Build history of the part. All positions in model axes, mm. A direction names the side the tool comes from. Give positions to 0.01 mm unless a question says otherwise; leave off trailing zeros. Loops run counter-clockwise (first coordinate to the right, second up) from the corner with the lowest first, then second, coordinate; pieces in that order, holes last.
1) Band-saw the part on B-B on z = -75. List the corners of the cut face in (x, y).
2) Two-plate mould, pull along Y, no slides. Class faces 1 (the flat face through (3, -2, -100)), 2 (the flat face through (2.96, 119.47, 83.25)), 3 (the flat face through (3, -150, 1)): +Y half, -Y half, draft (parallel to the pull), parting line (faces both ways), or undercut.
3) 3-axis set-ups, long thin cutter, end or side, ignore diameter. For faces 4 (the flat face through (2.96, 47.33, 27.95)), 5 (the flat face through (0, 2, 1)): which of +Z, -Z, +X, -X, +Y, -Y reach the whole face in a straight line?
4) Band-saw the part on A-A on x = 1.1. List the corners of the cut face in (y, z), then the cut area to 3 significant figures.
5) Wall check: line 1 (Z direction, x = 1.8, y = 38); line 2 (Y direction, x = 0.8, z = -15); line 3 (Z direction, x = 2.2, y = 129.5). Give the ranges that are in metal, low to high.
```python
from build123d import *

# Parameters (mm, degrees)
SKETCH_1_W      = 200
SKETCH_1_H      = 300
EXTRUDE_1_DEPTH = 6


with BuildPart() as part:
    # Эскиз1 → Бобышка-Вытянуть1 (new body)
    with BuildSketch(Plane(origin=(0, 0, 0), x_dir=(0, 0, -1), z_dir=(1, 0, 0))):
        Rectangle(SKETCH_1_W, SKETCH_1_H)
        Polygon((-91.932327425, 143.306818051), (-96.924629192, 139.978616874), (-69.18961938, 98.376102157), (-64.197317614, 101.704303335), align=None, mode=Mode.SUBTRACT)
        Polygon((-19.26660172, 23.491575667), (-14.274299954, 26.819776844), (-42.009309765, 68.422291561), (-47.001611531, 65.094090384), align=None, mode=Mode.SUBTRACT)
        Polygon((19.26660172, 23.491575667), (47.001611531, 65.094090384), (42.009309765, 68.422291561), (14.274299954, 26.819776844), align=None, mode=Mode.SUBTRACT)
        Polygon((96.924629192, 139.978616874), (69.18961938, 98.376102157), (64.197317614, 101.704303335), (91.932327425, 143.306818051), align=None, mode=Mode.SUBTRACT)
    extrude(amount=EXTRUDE_1_DEPTH)


solid = part.part
```
Findings below:
1. outline: (0, -150) - (6, -150) - (6, 107.09) - (0, 107.09) - close; (0, 117.91) - (6, 117.91) - (6, 150) - (0, 150) - close
2. face 1: draft
2. face 2: undercut
2. face 3: -Y half
3. face 4: +X, -X
3. face 5: +Z, -Z, -X, +Y, -Y
4. outline: (-150, -100) - (150, -100) - (150, 100) - (-150, 100) - close; hole (23.49, -19.27) - (65.09, -47) - (68.42, -42.01) - (26.82, -14.27) - close; hole (23.49, 19.27) - (26.82, 14.27) - (68.42, 42.01) - (65.09, 47) - close; hole (98.38, -69.19) - (139.98, -96.92) - (143.31, -91.93) - (101.7, -64.2) - close; hole (98.38, 69.19) - (101.7, 64.2) - (143.31, 91.93) - (139.98, 96.92) - close
4. area: 58,800 mm2
5. line 1: z = -100 to -28.94, -21.73 to 21.73, 28.94 to 100
5. line 2: y = -150 to 26.34, 27.91 to 150
5. line 3: z = -100 to -89.94, -82.73 to 82.73, 89.94 to 100
